Here's how the part is built. I have some questions about the finished solid (model axes, mm). Face numbers are marked on the shaded views. A direction names the side the tool comes from. Coordinates: 2 decimals unless noted, no trailing zeros. Write each loop counter-clockwise with the first axis right and the second up, starting at its lowest first coordinate (ties: lowest second). Pieces come first, ordered by that corner, then holes.
Item 1: For the marked faces 3 and 4, which set-ups out of +Z, -Z, +X, -X, +Y, -Y let a thin tool reach every point of the face, with its end or its side?
Item 2: If we section it at C-C (y = 5): Please give me the cut outline in (x, z), then the cut area to 3 significant figures.
Item 3: If we section it at A-A (x = 0): Please give me the cut outline in (y, z).
Item 4: If we section it at B-B (z = 3): Please give me the cut outline in (x, y), then the cut area to 3 significant figures.
Item 5: If we section it at D-D (y = 2): Please give me the cut outline in (x, z).
Item 6: We'd pull the mould along Z, two halves only. Please class the marked faces 1 and 2: +Z half, -Z half, draft (parallel to the pull), parting line (faces both ways), or undercut.
Item 7: If I drill on line 1 (Y direction, x = 0, z = -13); line 2 (Z direction, x = -4.5, y = 2.75); line 3 (X direction, y = 6.75, z = -9.5), over which ranges is the centre line in solid material (lowest first)?
Item 8: I'm going to push flat-ended pins straight in: pin 1 Ø1 at (x, y) = (-14, 9) entering from -Z; pin 2 Ø1.5 at (y, z) = (6, -6) entering from +X; pin 3 Ø5 at (y, z) = (2, 0.5) entering from +X; pin 4 Ø1 at (x, y) = (-9.5, 5) entering from +Z. Where does each tip first touch, or does it pass through?
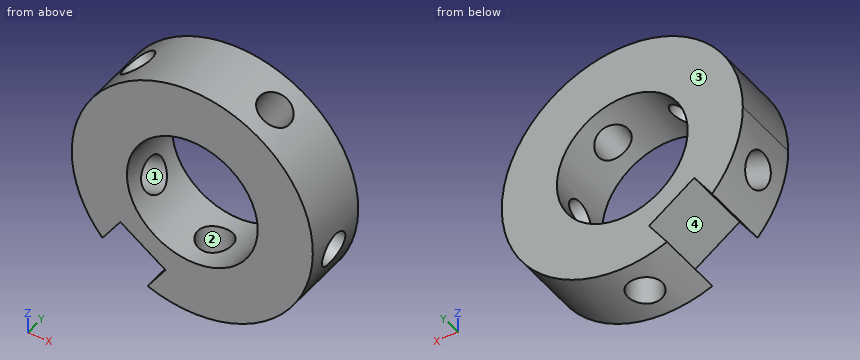
Autodesk Inventor part; units mm, degrees
ref_plane "Work Plane13" through (0, 0, 0) normal (0, 0, 1) x (0, 1, 0)
ref_plane "Work Plane14" through (0, 0, 0) normal (0.9397, 0, 0.342) x (0, 1, 0)
ref_plane "Work Plane15" through (0, 0, 0) normal (0.6428, 0, -0.766) x (0, 1, 0)
sketch "Sketch1" plane through (0, 0, 0) normal (0, 1, 0) x (-1, 0, 0)
  circle A0 centre (0, 0) radius 17.5
  dimension "d0" = 35
extrude "Extrusion1" add sketch "Sketch1" along normal blind 10
sketch "Sketch2" plane through (0, 10, 0) normal (0, 1, 0) x (1, 0, 0)
  circle A0 centre (0, 0) radius 9.5
  dimension "d3" = 19
extrude "Extrusion2" cut sketch "Sketch2" against normal through all
ref_plane "Work Plane13" through (0, 0, 0) normal (0, 0, 1) x (0, 1, 0)
sketch "Sketch11" plane through (0, 0, 0) normal (0, 0, 1) x (0, 1, 0)
  circle A0 centre (5, 0) radius 2.5
  point P0 (0, 0)
  dimension "d52" = 5
hole "Hole5" at (0, 5, 0) direction (0, 0, -1) diameter 5 end through all
ref_plane "Work Plane14" through (0, 0, 0) normal (0.9397, 0, 0.342) x (0, 1, 0)
sketch "Sketch12" plane through (0, 0, 0) normal (0.9397, 0, 0.342) x (0, 1, 0)
  circle A0 centre (5, 0) radius 2.5
  point P0 (0, 0)
  dimension "d61" = 5
hole "Hole6" at (0, 5, 0) direction (-0.9397, 0, -0.342) diameter 5 end through all
ref_plane "Work Plane15" through (0, 0, 0) normal (0.6428, 0, -0.766) x (0, 1, 0)
sketch "Sketch13" plane through (0, 0, 0) normal (0.6428, 0, -0.766) x (0, 1, 0)
  circle A0 centre (5, 0) radius 2.5
  point P0 (0, 0)
  dimension "d70" = 5
hole "Hole7" at (0, 5, 0) direction (-0.6428, 0, 0.766) diameter 5 end through all
ref_plane "Work Plane16" through (0, 0, 0) normal (-0.5, 0, -0.866) x (0, 1, 0)
sketch "Sketch14" plane through (0, 0, 0) normal (-0.5, 0, -0.866) x (0, 1, 0)
  circle A0 centre (5, 0) radius 2.5
  point P0 (0, 0)
  dimension "d79" = 5
hole "Hole8" at (0, 5, 0) direction (0.5, 0, 0.866) diameter 5 end through all
ref_plane "Work Plane17" through (0, 0, 0) normal (-0.9848, 0, 0.1736) x (0, 1, 0)
sketch "Sketch15" plane through (0, 0, 0) normal (-0.9848, 0, 0.1736) x (0, 1, 0)
  circle A0 centre (5, 0) radius 2.5
  point P0 (0, 0)
  dimension "d88" = 5
hole "Hole9" at (0, 5, 0) direction (0.9848, 0, -0.1736) diameter 5 end through all
ref_plane "Work Plane21" through (-10.0376, 0, -14.3352) normal (0.5736, 0, 0.8192) x (0, 1, 0)
ref_plane "Work Plane20" through (0, 0, 0) normal (0.5736, 0, 0.8192) x (0, 1, 0)
sketch "Sketch16" plane through (-10.0376, 0, -14.3352) normal (0.5736, 0, 0.8192) x (0, 1, 0)
  line L0 (10, 4) -> (0, 4)
  line L1 (0, 4) -> (0, -4)
  line L2 (0, -4) -> (10, -4)
  line L3 (10, -4) -> (10, 4)
  line L4 (0, 17.5) -> (0, -17.5)
  line L5 (18.3389, 0) -> (-7, 0) construction
  point P0 (0, 0)
  dimension "d100" = 8
  dimension "d107" = 4
  dimension "d108" = 10
extrude "Extrusion4" cut sketch "Sketch16" along normal blind 5
sketch "Sketch17" plane through (0, 0, 0) normal (0, -1, 0) x (1, 0, 0)
  line L0 (0, 0) -> (-16.3488, -23.3485) construction
  line L1 (-10.4463, -7.9451) -> (-13.0485, -11.6614) construction
  line L2 (-6.4953, -16.25) -> (-3.8931, -12.5337) construction
  line L3 (-3.8931, -12.5337) -> (-6.4953, -16.25)
  arc A0 (-6.4953, -16.25) -> (-13.0485, -11.6614) centre (0, 0) ccw
  line L4 (-13.0485, -11.6614) -> (-10.4463, -7.9451)
  line L5 (-10.4463, -7.9451) -> (-3.8931, -12.5337)
  circle A1 centre (0, 0) radius 9.5
  point P0 (-10.0012, -14.2832)
  dimension "d114" = 26.426
  dimension "d115" = 13.213
equation "\"d107\" = 0.5 * d100"
properties part number "sprzeglo_04"
Answer list:
1. face 3: +Z, -Z, +X, -X, +Y
1. face 4: +Y, -Y
2. outline: (-17.13, -3.57) - (-9.47, -0.79) arc R9.5 cw to (-7.81, 5.41) - (-13.05, 11.66) arc R17.5 ccw to start; (-15.42, -8.27) arc R17.5 ccw to (-13.05, -11.66) - (-10.45, -7.94) - (-3.89, -12.53) - (-6.5, -16.25) arc R17.5 ccw to (-2.5, -17.32) - (-2.5, -9.17) arc R9.5 cw to (-7.76, -5.48) - close; (-9.22, 14.88) - (-3.98, 8.63) arc R9.5 cw to (2.42, 9.19) - (6.5, 16.25) arc R17.5 ccw to start; (2.5, -17.32) arc R17.5 ccw to (16.62, -5.47) - (8.59, -4.05) arc R9.5 cw to (2.5, -9.17) - close; (6.75, 6.69) arc R9.5 cw to (9.46, 0.87) - (17.49, -0.55) arc R17.5 ccw to (10.83, 13.75) - close
2. area: 439 mm2
3. outline: (0, -17.5) - (2.5, -17.5) - (2.5, -9.5) - (0, -9.5) - close; (0, 9.5) - (10, 9.5) - (10, 17.5) - (0, 17.5) - close; (7.5, -17.5) - (10, -17.5) - (10, -9.5) - (7.5, -9.5) - close
4. outline: (-17.24, 0) - (-9.01, 0) - (-9.01, 10) - (-17.24, 10) - close; (9.01, 0) - (17.24, 0) - (17.24, 10) - (9.01, 10) - close
4. area: 165 mm2
5. outline: (-13.05, -11.66) - (-10.45, -7.94) - (-3.89, -12.53) - (-6.5, -16.25) arc R17.5 ccw (long way) to start; hole circle Ø19 at (0, 0)
6. face 1: undercut
6. face 2: draft
7. line 1: y = 0 to 2.5, 7.5 to 10
7. line 2: z = -16.91 to -13.4, -12.11 to -8.37, 8.37 to 16.91
7. line 3: x = -14.7 to -11.54, -8.22 to -1.79, 1.79 to 14.7
8. pin 1: stops at z = -11.14
8. pin 2: stops at x = 16.69
8. pin 3: stops at x = 17.5
8. pin 4: stops at z = 15.01
